Model file for the job. Use its own axes, mm. Face numbers are marked on the shaded views. A direction names the side the tool comes from. Round coordinates to 2 decimals unless told otherwise and drop trailing zeros. Order: outer loops, then holes, each group sorted by start corner. A loop starts at its lowest first (then second) coordinate and runs counter-clockwise, first axis right, second up. Notation, with made-up numbers: (-24.5, -38.5) - (13.5, -38.5) arc R21 cw to (13.5, -13.5) - close; hole circle Ø11 at (9, 83.25). An arc over 180 degrees is marked (long way). Use one line per item in the form item = value.
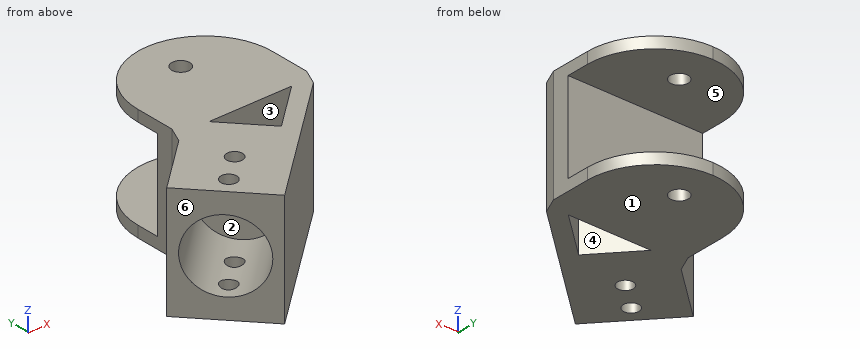
from build123d import *

# Parameters (mm, degrees)
BOSS_EXTRUDE4_DEPTH = 50
SKETCH6_W           = 59.76747767
SKETCH6_H           = 50
BOSS_EXTRUDE5_DEPTH = 52
SKETCH7_W           = 50
SKETCH7_H           = 40
CUT_EXTRUDE2_DEPTH  = 50
SKETCH9_R           = 16
CUT_EXTRUDE3_DEPTH  = 39
SKETCH10_W          = 59.76747767
SKETCH10_H          = 40
CUT_EXTRUDE4_DEPTH  = 50
CUT_EXTRUDE5_REACH  = 133.427
SKETCH11_R          = 4
CUT_EXTRUDE6_REACH  = 133.427
SKETCH12_R          = 3.5
FILLET2_R           = 30
SKETCH17_W          = 59.76747767
SKETCH17_H          = 40
BOSS_EXTRUDE8_DEPTH = 10
CUT_EXTRUDE8_DEPTH  = 50


with BuildPart() as part:
    # Sketch5 → Boss-Extrude4 (new body)
    with BuildSketch(Plane.XY):
        Polygon((0, 53.833769989), (59.76747767, 53.833769989), (-37.490513215, -33.76845977), (-64.260925192, -4.047338616), align=None)
    extrude(amount=BOSS_EXTRUDE4_DEPTH)

    # Sketch6 → Boss-Extrude5 (add)
    with BuildSketch(Plane(origin=(0, 53.833769989, 0), x_dir=(1, 0, 0), z_dir=(0, 1, 0))):
        with Locations((29.883738835, -25)):
            Rectangle(SKETCH6_W, SKETCH6_H)
    extrude(amount=BOSS_EXTRUDE5_DEPTH)

    # Sketch7 → Cut-Extrude2 (cut)
    with BuildSketch(Plane(origin=(-37.490513215, -33.768459769, 0), x_dir=(0, 0, 1), z_dir=(-0.7430280288371722, -0.6692602994069995, 0))):
        with Locations((25, 20)):
            Rectangle(SKETCH7_W, SKETCH7_H)
    extrude(amount=-CUT_EXTRUDE2_DEPTH, mode=Mode.SUBTRACT)

    # Sketch9 → Cut-Extrude3 (cut)
    with BuildSketch(Plane(origin=(-0.339111773, -0.305444799, 0), x_dir=(0, 0, 1), z_dir=(-0.743028028837172, -0.6692602994069997, 0))):
        with Locations(Location((25, 20, 0), (0, 0, 270))):
            Circle(SKETCH9_R)
    extrude(amount=-CUT_EXTRUDE3_DEPTH, mode=Mode.SUBTRACT)

    # Sketch10 → Cut-Extrude4 (cut)
    with BuildSketch(Plane(origin=(0, 105.833769989, 0), x_dir=(1, 0, 0), z_dir=(0, 1, 0))):
        with Locations((29.883738835, -25)):
            Rectangle(SKETCH10_W, SKETCH10_H)
    extrude(amount=-CUT_EXTRUDE4_DEPTH, mode=Mode.SUBTRACT)

    # Cut-Extrude5: up to this face of the body (flat: up to its plane)
    cut_extrude5_end = Plane(part.part.faces().sort_by_distance((21.675181221, 59.791215604, 0))[0])
    # Sketch11 → Cut-Extrude5 (cut, up to the picked face)
    with BuildSketch(Plane.XY.offset(50), mode=Mode.PRIVATE) as cut_extrude5_sk1:
        with Locations(Location((29.76747767, 88.333769989, 0), (0, 0, 180))):
            Circle(SKETCH11_R)
    cut_extrude5_tool1 = split(extrude(cut_extrude5_sk1.sketch, amount=-CUT_EXTRUDE5_REACH, mode=Mode.PRIVATE), bisect_by=cut_extrude5_end, keep=Keep.BOTH, mode=Mode.PRIVATE)
    add(cut_extrude5_tool1.solids().sort_by(Axis((29.767478, 88.33377, 50), (0, 0, -1)))[0], mode=Mode.SUBTRACT)

    # Cut-Extrude6: up to this face of the body (flat: up to its plane)
    cut_extrude6_end = Plane(part.part.faces().sort_by_distance((21.599927582, 59.525786489, 0))[0])
    # Sketch12 → Cut-Extrude6 (cut, up to the picked face)
    with BuildSketch(Plane.XY.offset(50), mode=Mode.PRIVATE) as cut_extrude6_sk1:
        with Locations((3.855725401, 30.389814462)):
            Circle(SKETCH12_R)
    cut_extrude6_tool1 = split(extrude(cut_extrude6_sk1.sketch, amount=-CUT_EXTRUDE6_REACH, mode=Mode.PRIVATE), bisect_by=cut_extrude6_end, keep=Keep.BOTH, mode=Mode.PRIVATE)
    # Sketch12 → Cut-Extrude6 (cut, up to the picked face)
    with BuildSketch(Plane.XY.offset(50), mode=Mode.PRIVATE) as cut_extrude6_sk2:
        with Locations((-7.534894281, 20.130054072)):
            Circle(SKETCH12_R)
    cut_extrude6_tool2 = split(extrude(cut_extrude6_sk2.sketch, amount=-CUT_EXTRUDE6_REACH, mode=Mode.PRIVATE), bisect_by=cut_extrude6_end, keep=Keep.BOTH, mode=Mode.PRIVATE)
    add(cut_extrude6_tool1.solids().sort_by(Axis((3.855725, 30.389814, 50), (0, 0, -1)))[0], mode=Mode.SUBTRACT)
    add(cut_extrude6_tool2.solids().sort_by(Axis((-7.534894, 20.130054, 50), (0, 0, -1)))[0], mode=Mode.SUBTRACT)

    # Fillet2
    # the kernel refuses this fillet: 30 mm, written as the material it takes off along each edge
    with BuildSketch(Plane(origin=(59.76747767, 105.833769989, 125), x_dir=(0, -1, 0), z_dir=(0, 0, -1)), Plane(origin=(0, 105.833769989, -30), x_dir=(0, -1, 0), z_dir=(0, 0, 1)), Plane(origin=(59.76747767, 105.833769989, 80), x_dir=(0, -1, 0), z_dir=(0, 0, -1))) as fillet2_piece_1:
        with BuildLine():
            CenterArc((FILLET2_R, FILLET2_R), FILLET2_R, 180, 90)
            Line((0, FILLET2_R), (0, 0))
            Line((0, 0), (FILLET2_R, 0))
        make_face()
    extrude(amount=155, mode=Mode.SUBTRACT)
    with BuildSketch(Plane(origin=(0, 105.833769989, -75), x_dir=(1, 0, 0), z_dir=(0, 0, 1))) as fillet2_piece_2:
        with BuildLine():
            CenterArc((FILLET2_R, -FILLET2_R), FILLET2_R, 90, 90)
            Line((0, -FILLET2_R), (0, 0))
            Line((0, 0), (FILLET2_R, 0))
        make_face()
    extrude(amount=155, mode=Mode.SUBTRACT)

    # Sketch17 → Boss-Extrude8 (add)
    with BuildSketch(Plane(origin=(0, 55.833769989, 0), x_dir=(1, 0, 0), z_dir=(0, 1, 0))):
        with Locations((29.883738835, -25)):
            Rectangle(SKETCH17_W, SKETCH17_H)
    extrude(amount=BOSS_EXTRUDE8_DEPTH)

    # Chamfer5
    # the kernel refuses this chamfer: 10 mm, written as the material it adds along each edge
    with BuildSketch(Plane(origin=(0, 53.833769989, 0), x_dir=(0.03375152736497673, 0.9994302548955236, 0), z_dir=(0, 0, 1))) as chamfer5_piece_1:
        with BuildLine():
            Line((4.819419462, 0), (-3.459685747, 3.355201705))
            Line((-3.459685747, 3.355201705), (-3.603688974, 3.216410241))
            ThreePointArc((-3.603688974, 3.216410241), (-1.815286192, 1.595249898), (-0.144003227, -0.138791464))
            Line((-0.144003227, -0.138791464), (0.006750305, -0.199886051))
            ThreePointArc((0.006750305, -0.199886051), (2.413714978, -0.118601005), (4.826169768, -0.199886051))
            Line((4.826169768, -0.199886051), (4.819419462, 0))
        make_face()
    extrude(amount=50)

    # Chamfer6
    # the kernel refuses this chamfer: 10 mm, written as the material it takes off along each edge
    with BuildSketch(Plane(origin=(59.76747767, 53.833769989, -12.048548655), x_dir=(0.03375152736497822, 0.9994302548955234, 0), z_dir=(0, 0, 1))) as chamfer6_piece_1:
        with BuildLine():
            Line((4.819419462, 0), (-3.459685747, 3.355201705))
            Line((-3.459685747, 3.355201705), (-3.603688974, 3.216410241))
            ThreePointArc((-3.603688974, 3.216410241), (-1.815286192, 1.595249898), (-0.144003227, -0.138791464))
            Line((-0.144003227, -0.138791464), (0.006750305, -0.199886051))
            ThreePointArc((0.006750305, -0.199886051), (2.413714978, -0.118601005), (4.826169768, -0.199886051))
            Line((4.826169768, -0.199886051), (4.819419462, 0))
        make_face()
    extrude(amount=74.097097311, mode=Mode.SUBTRACT)

    # Sketch18 → Cut-Extrude8 (cut)
    with BuildSketch(Plane(origin=(0, 0, 0), x_dir=(-1, 0, 0), z_dir=(0, 0, -1))):
        Polygon((-29.160349369, 35.686223292), (-49.412180648, 53.927455304), (-12.730104581, 53.927455304), align=None)
    extrude(amount=-CUT_EXTRUDE8_DEPTH, mode=Mode.SUBTRACT)


solid = part.part
(1) Slice it at A-A on z = 16. Give the cut face in (x, y), then the cut area to 3 significant figures.
Report:
outline = (-27.11, 29.42) - (-22.58, 24.38) - (6.4, 50.49) - (24.11, 30.83) - (-4.87, 4.73) - (-0.34, -0.31) - (56.46, 50.85) - (59.77, 58.29) - (59.77, 65.83) - (0, 65.83) - (0, 58.29) - (-3.31, 50.85) - close; hole (12.73, 53.93) - (29.16, 35.69) - (49.41, 53.93) - close
area = 1,700 mm2
(2) Pull direction Z, two halves, no side cores. Call the marked faces 1, 2 and 3: released by +Z, released by -Z, zero draft, split by the parting line, or undercut.
Report:
face_1 = released by -Z
face_2 = undercut
face_3 = zero draft
(3) Slice it at B-B on y = 79. Give the cut face in (x, z).
Report:
outline = (0.17, 0) - (59.6, 0) - (59.6, 5) - (0.17, 5) - close; (0.17, 45) - (59.6, 45) - (59.6, 50) - (0.17, 50) - close
(4) Slice it at C-C on y = 49. Count the separate pieces of the cut face and the enclosed holes in it, then the cut area to 3 significant figures.
Report:
separate_pieces = 2
enclosed_holes = 1
area = 1,540 mm2
(5) Pin check, flat tips, straight feed: pin 1 (1 mm diameter, centred on y = 28, z = 27.5, fed in from +X); pin 2 (4 mm diameter, centred on x = -7.53, y = 20.13, fed in from +Z); pin 3 (5 mm diameter, centred on y = 30, z = 44.5, fed in from -X); pin 4 (5 mm diameter, centred on y = 14, z = 5.5, fed in from -X). Stop position of each tip, or through.
Report:
pin_1 = 31.64
pin_2 = through
pin_3 = -27.11
pin_4 = -15.48
(6) Slice it at D-D on x = 52. Give the cut face in (y, z).
Report:
outline = (46.84, 0) - (95.98, 0) - (95.98, 5) - (65.83, 5) - (65.83, 45) - (95.98, 45) - (95.98, 50) - (46.84, 50) - close
(7) Probe probe 1 along Y at (x, z) = (16, 20); probe 2 along Z at (x, y) = (56, 75); probe 3 along X at (y, z) = (39.5, 36). List the from-to ranges inside material, lowest first. Write a range as [from, to].
Report:
probe_1 = [14.41, 20.87], [39.83, 50.3], [53.93, 65.83]
probe_2 = [0, 5], [45, 50]
probe_3 = [-15.91, -3.39], [16.3, 25.73], [33.39, 43.85]
(8) Tool access for the marked faces 4, 5 and 6: list every direction of +Z, -Z, +X, -X, +Y, -Y with a clear straight run to the whole face (end or side of a thin tool).
Report:
face_4 = +Z, -Z
face_5 = +X, -X, +Y
face_6 = +Z, -Z, -X, -Y
